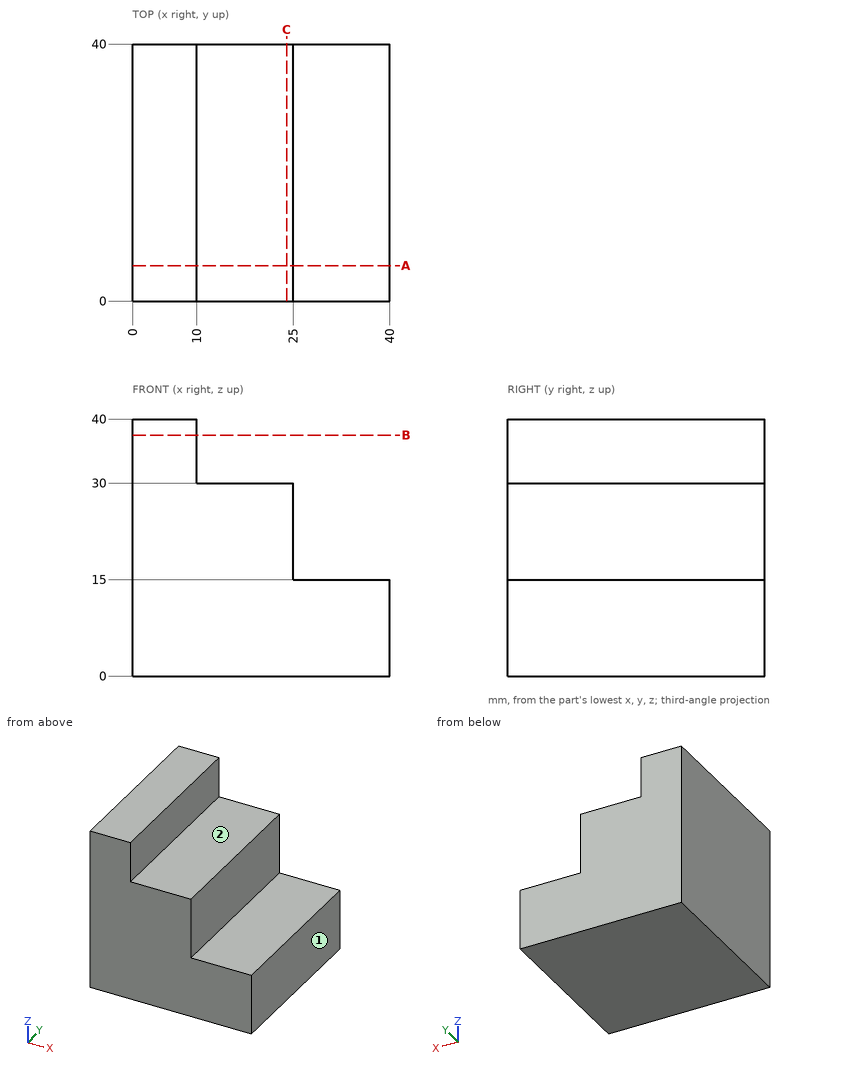
Drawing for the job (mm, zero at the part's lowest x, y, z). A direction names the side the tool comes from. Coordinates: 2 decimals unless noted, no trailing zeros. Order: outer loops, then holes, each group sorted by start corner. A loop starts at its lowest first (then second) coordinate and runs counter-clockwise, first axis right, second up.
Item 1: Band-saw the part on C-C on x = 24. List the corners of the cut face in (y, z).
Check sheet entries:
outline: (0, 0) - (40, 0) - (40, 30) - (0, 30) - close
Item 2: Drill centre lines: L1, parallel to Z at x = 27, y = 36.5; L2, parallel to Z at x = 22, y = 4; L3, parallel to X at y = 6, z = 35. Where is each one in solid material? Low to high.
Check sheet entries:
L1: z = 0 to 15
L2: z = 0 to 30
L3: x = 0 to 10
Item 3: Band-saw the part on B-B on z = 37.5. List the corners of the cut face in (x, y), plus the area to 3 significant figures.
Check sheet entries:
outline: (0, 0) - (10, 0) - (10, 40) - (0, 40) - close
area: 400 mm2
Item 4: Band-saw the part on A-A on y = 5.5. List the corners of the cut face in (x, z), plus the area to 4 significant figures.
Check sheet entries:
outline: (0, 0) - (40, 0) - (40, 15) - (25, 15) - (25, 30) - (10, 30) - (10, 40) - (0, 40) - close
area: 1,075 mm2
Item 5: 3-axis set-ups, long thin cutter, end or side, ignore diameter. For the marked faces 1 and 2: which of +Z, -Z, +X, -X, +Y, -Y reach the whole face in a straight line?
Check sheet entries:
face 1: +Z, -Z, +X, +Y, -Y
face 2: +Z, +X, +Y, -Y
Item 6: Pin check, flat tips, straight feed: pin 1 Ø4.5 at (x, y) = (30, 29.5) entering from +Z; pin 2 Ø4.5 at (y, z) = (19.5, 19.5) entering from +X; pin 3 Ø7.5 at (x, y) = (16.5, 22.5) entering from +Z. Stop position of each tip, or through.
Check sheet entries:
pin 1: stops at z = 15
pin 2: stops at x = 25
pin 3: stops at z = 30
